```python
from build123d import *

# Parameters (mm, degrees)
SKETCH1_R               = 5.5
BLOCO_DEPTH             = 11
SKETCH2_W               = 11
SKETCH2_H               = 15
RASGOS_LATERAIS_DEPTH   = 26
SKETCH3_R               = 1.75
FUROS_DE_FIXA_O_4_DEPTH = 38.379807383


with BuildPart() as part:
    # Sketch1 → Bloco (new, symmetric)
    with BuildSketch(Plane.XY):
        with BuildLine():
            Line((-6.947113934, 24.897714569), (-24.5, 0))
            Line((-24.5, 0), (24.5, 0))
            Line((24.5, 0), (6.947113934, 24.897714569))
            ThreePointArc((6.947113934, 24.897714569), (0, 28.5), (-6.947113934, 24.897714569))
        make_face()
        with Locations((0, 20)):
            Circle(SKETCH1_R, mode=Mode.SUBTRACT)
    extrude(amount=BLOCO_DEPTH, both=True)

    # Sketch2 → Rasgos Laterais (cut)
    with BuildSketch(Plane(origin=(0, 28.5, 0), x_dir=(1, 0, 0), z_dir=(0, 1, 0))):
        with Locations((19, 0)):
            Rectangle(SKETCH2_W, SKETCH2_H)
        with Locations((-19, 0)):
            Rectangle(SKETCH2_W, SKETCH2_H)
    extrude(amount=-RASGOS_LATERAIS_DEPTH, mode=Mode.SUBTRACT)

    # Sketch3 → Furos de Fixação Ø4 (cut, through all)
    with BuildSketch(Plane(origin=(0, 2.5, 0), x_dir=(1, 0, 0), z_dir=(0, 1, 0))):
        with Locations(Location((20, 0, 0), (0, 0, 270))):
            Circle(SKETCH3_R)
        with Locations(Location((-20, 0, 0), (0, 0, 90))):
            Circle(SKETCH3_R)
    extrude(amount=-FUROS_DE_FIXA_O_4_DEPTH, mode=Mode.SUBTRACT)


solid = part.part
```
Here's how the part is built. I have some questions about the finished solid (model axes, mm). A direction names the side the tool comes from. Coordinates: 2 decimals unless noted, no trailing zeros. Order: outer loops, then holes, each group sorted by start corner. A loop starts at its lowest first (then second) coordinate and runs counter-clockwise, first axis right, second up.
1) Will these pins go through, and if not, where does the flat tip stop? pin 1 (3 mm diameter, centred on x = -17.5, z = 3.5, fed in from +Y); pin 2 (5.5 mm diameter, centred on x = -20, z = 0, fed in from -Y); pin 3 (6 mm diameter, centred on y = 9.5, z = 3, fed in from -X); pin 4 (10.5 mm diameter, centred on y = 12.5, z = -0.5, fed in from +X).
2) I need wall thicknesses on line 1 (Y direction, x = 0, z = 2); line 2 (Z direction, x = -20, y = 1.9); line 3 (X direction, y = 1.9, z = 0). Which ranges of each line are inside material? Lowest first, please.
3) Imagine slicing it at D-D on z = 2.25. List the corners of the cut face in (x, y) for me, and give its area (3 significant figures).
4) Imagine slicing it at C-C on y = 20.5. List the corners of the cut face in (x, z) for me.
5) Imagine slicing it at A-A on z = 0. List the corners of the cut face in (x, y) for me.
6) Imagine slicing it at B-B on x = 0. List the corners of the cut face in (y, z) for me, and give its area (3 significant figures).
7) We'd pull the mould along Z, two halves only. Please class faces 4 (the face through (21.735, 1.268, -0.228)), 5 (the face through (-11.7, 18.156, 0.154)), 6 (the face through (0, 11, 11)): +Z half, -Z half, draft (parallel to the pull), parting line (faces both ways), or undercut.
8) Which directions (+Z, -Z, +X, -X, +Y, -Y) give clear straight access to the entire face, cutting with the end or side of a thin tool? Please do faces 1 (the face through (18, 2.5, 0)), 2 (the face through (-13.5, 9, 0)), 3 (the face through (0, 0, 0)).
Response values:
1. pin 1: stops at y = 2.5
1. pin 2: stops at y = 0
1. pin 3: stops at x = -13.5
1. pin 4: stops at x = 13.5
2. line 1: y = 0 to 14.5, 25.5 to 28.5
2. line 2: z = -11 to -1.75, 1.75 to 11
2. line 3: x = -23.16 to -21.75, -18.25 to 18.25, 21.75 to 23.16
3. outline: (-24.5, 0) - (24.5, 0) - (22.74, 2.5) - (13.5, 2.5) - (13.5, 15.6) - (6.95, 24.9) arc R8.5 ccw to (-6.95, 24.9) - (-13.5, 15.6) - (-13.5, 2.5) - (-22.74, 2.5) - close; hole circle Ø11 at (0, 20)
3. area: 602 mm2
4. outline: (-10.05, -11) - (-5.48, -11) - (-5.48, 11) - (-10.05, 11) - close; (5.48, -11) - (10.05, -11) - (10.05, 11) - (5.48, 11) - close
5. outline: (-24.5, 0) - (-21.75, 0) - (-21.75, 2.5) - (-22.74, 2.5) - close; (-18.25, 0) - (18.25, 0) - (18.25, 2.5) - (13.5, 2.5) - (13.5, 15.6) - (6.95, 24.9) arc R8.5 ccw to (-6.95, 24.9) - (-13.5, 15.6) - (-13.5, 2.5) - (-18.25, 2.5) - close; (21.75, 0) - (24.5, 0) - (22.74, 2.5) - (21.75, 2.5) - close; hole circle Ø11 at (0, 20)
6. outline: (0, -11) - (14.5, -11) - (14.5, 11) - (0, 11) - close; (25.5, -11) - (28.5, -11) - (28.5, 11) - (25.5, 11) - close
6. area: 385 mm2
7. face 4: undercut
7. face 5: draft
7. face 6: +Z half
8. face 1: +X, +Y
8. face 2: -X, +Y
8. face 3: +Z, -Z, +X, -X, -Y
